Check sheet for the modelled part. Datum: model origin and axes. Units: mm. Face numbers are marked on the shaded views. A direction names the side the tool comes from. Round coordinates to 2 decimals unless told otherwise and drop trailing zeros. Write each loop counter-clockwise with the first axis right and the second up, starting at its lowest first coordinate (ties: lowest second). Pieces come first, ordered by that corner, then holes. Notation, with made-up numbers: (-26, -7.75) -> (-12, -7.75) arc R27 ccw to (-12, 28.25) -> close; hole circle Ø8 at (40, -25). An arc over 180 degrees is marked (long way). Write item = value, one per line.
from build123d import *

# Parameters (mm, degrees)
SKETCH_1_W            = 140
SKETCH_1_H            = 33
EXTRUDE_1_DEPTH       = 3
HOLE_WIZARD_1_D       = 3.5
SKETCH_5_W            = 10
SKETCH_5_H            = 33
EXTRUDE_2_DEPTH       = 31
SKETCH_6_W            = 140
SKETCH_6_H            = 33
EXTRUDE_3_DEPTH       = 3
HOLE_WIZARD_2_D       = 4
HOLE_WIZARD_2_DEPTH   = 3
EXTRUDE_7_DEPTH       = 3
MIRROR_4_COPY_1_DEPTH = 3
EXTRUDE_8_DEPTH       = 3
SKETCH_12_W           = 10
SKETCH_12_H           = 31
CUT_EXTRUDE_1_DEPTH   = 85.528101836
SKETCH_14_W           = 18
SKETCH_14_H           = 3.3
CUT_EXTRUDE_3_DEPTH   = 3
SKETCH_17_W           = 30
SKETCH_17_H           = 15
CUT_EXTRUDE_5_DEPTH   = 5
SKETCH_22_W           = 15
SKETCH_22_H           = 15.5
CUT_EXTRUDE_6_DEPTH   = 3
SKETCH_23_W           = 93
SKETCH_23_H           = 20
CUT_EXTRUDE_7_DEPTH   = 13.5
SKETCH_24_W           = 59
SKETCH_24_H           = 14
CUT_EXTRUDE_8_DEPTH   = 3
SKETCH_26_W           = 59
SKETCH_26_H           = 3
EXTRUDE_9_DEPTH       = 33
SKETCH_27_W           = 1.5
SKETCH_27_H           = 28.5
CUT_EXTRUDE_9_DEPTH   = 3
SKETCH_28_W           = 10
SKETCH_28_H           = 3
EXTRUDE_10_DEPTH      = 3
SKETCH_29_W           = 10
SKETCH_29_H           = 15
CUT_EXTRUDE_10_DEPTH  = 3
SKETCH_30_W           = 4
SKETCH_30_H           = 11
EXTRUDE_11_DEPTH      = 3
CUT_EXTRUDE_11_REACH  = 77.507
SKETCH_31_W           = 7
SKETCH_31_H           = 11
SKETCH_35_W           = 5
SKETCH_35_H           = 11
CUT_EXTRUDE_12_DEPTH  = 13.5
HOLE_WIZARD_3_D       = 3.3
HOLE_WIZARD_3_DEPTH   = 3


with BuildPart() as part:
    # 草图1 → 凸台-拉伸1 (new body)
    with BuildSketch(Plane(origin=(0, 0, 0), x_dir=(1, 0, 0), z_dir=(0, 1, 0))):
        Rectangle(SKETCH_1_W, SKETCH_1_H)
    extrude(amount=EXTRUDE_1_DEPTH)

    # 孔1 (through all)
    with Locations(Plane(origin=(0, 3, 0), x_dir=(1, 0, 0), z_dir=(0, 1, 0))):
        with Locations((-66.5, 13), (-12.5, 13), (-12.5, -13), (-66.5, -13)):
            hole_wizard_1 = Hole(HOLE_WIZARD_1_D / 2)

    # 镜向1: 孔1 across plane
    add(hole_wizard_1.mirror(Plane.ZY), mode=Mode.SUBTRACT)

    # 草图5 → 凸台-拉伸2 (add)
    with BuildSketch(Plane.XZ):
        with Locations((-44.5, 0)):
            Rectangle(SKETCH_5_W, SKETCH_5_H)
        with Locations((-34.5, 0)):
            Rectangle(SKETCH_5_W, SKETCH_5_H)
        with Locations((34.5, 0)):
            Rectangle(SKETCH_5_W, SKETCH_5_H)
        with Locations((44.5, 0)):
            Rectangle(SKETCH_5_W, SKETCH_5_H)
    extrude(amount=EXTRUDE_2_DEPTH)

    # 草图6 → 凸台-拉伸3 (add)
    with BuildSketch(Plane.XZ.offset(31)):
        Rectangle(SKETCH_6_W, SKETCH_6_H)
    extrude(amount=EXTRUDE_3_DEPTH)

    # 孔2
    with Locations(Plane(origin=(0, -34, 0), x_dir=(-1, 0, 0), z_dir=(0, -1, 0))):
        with Locations((57, 0), (22, 0)):
            hole_wizard_2 = Hole(HOLE_WIZARD_2_D / 2, depth=HOLE_WIZARD_2_DEPTH)

    # 镜向2: 孔2 across plane
    add(hole_wizard_2.mirror(Plane.ZY), mode=Mode.SUBTRACT)

    # 草图10 → 凸台-拉伸7 (add)
    with BuildSketch(Plane.XY.offset(16.5)):
        Polygon((-61.709614661, 0), (-49.5, -15.5), (-49.5, -9.231659865), align=None)
        Polygon((-61.709614661, 0), (-49.5, -9.231659865), (-56.771936106, 0), align=None)
        Polygon((-49.5, -15.5), (-70, -31), (-61.709614661, -31), (-49.5, -21.768340135), align=None)
    extrude_7 = extrude(amount=-EXTRUDE_7_DEPTH)

    # 镜向3: 凸台-拉伸7 across plane
    add(extrude_7.mirror(Plane.XY))

    # 镜向4: 凸台-拉伸7 across plane
    add(extrude_7.mirror(Plane.ZY))

    # 镜向4 copy 1 sketch → 镜向4 copy 1 (add)
    with BuildSketch(Plane(origin=(0, 0, -16.5), x_dir=(-1, 0, 0), z_dir=(0, 0, -1))):
        Polygon((-61.709614661, 0), (-49.5, -15.5), (-49.5, -9.231659865), align=None)
        Polygon((-61.709614661, 0), (-49.5, -9.231659865), (-56.771936106, 0), align=None)
        Polygon((-49.5, -15.5), (-70, -31), (-61.709614661, -31), (-49.5, -21.768340135), align=None)
    extrude(amount=-MIRROR_4_COPY_1_DEPTH)

    # 草图11 → 凸台-拉伸8 (add)
    with BuildSketch(Plane.XY.offset(16.5)):
        Polygon((-1.380422804, -1.450613794), (-29.5, -31), (-26.739154392, -31), (0, -2.901227588), align=None)
        Polygon((-29.5, -26.648158618), (-29.5, -31), (-1.380422804, -1.450613794), (0, 0), (-4.141268412, 0), align=None)
        Polygon((0, 0), (-1.380422804, -1.450613794), (0, -2.901227588), (1.380422804, -1.450613794), align=None)
        Polygon((1.380422804, -1.450613794), (0, -2.901227588), (26.739154392, -31), (29.5, -31), align=None)
        Polygon((4.141268412, 0), (0, 0), (1.380422804, -1.450613794), (29.5, -31), (29.5, -26.648158618), align=None)
    extrude_8 = extrude(amount=-EXTRUDE_8_DEPTH)

    # 镜向5: 凸台-拉伸8 across plane
    add(extrude_8.mirror(Plane.XY))

    # 草图12 → 切除-拉伸1 (cut, through all)
    with BuildSketch(Plane.XY.offset(16.5)):
        with Locations((-39.5, -15.5)):
            Rectangle(SKETCH_12_W, SKETCH_12_H)
    cut_extrude_1 = extrude(amount=-CUT_EXTRUDE_1_DEPTH, mode=Mode.SUBTRACT)

    # 镜向6: 切除-拉伸1 across plane
    add(cut_extrude_1.mirror(Plane.ZY), mode=Mode.SUBTRACT)

    # 草图14 → 切除-拉伸3 (cut)
    with BuildSketch(Plane(origin=(0, -31, 0), x_dir=(1, 0, 0), z_dir=(0, 1, 0))):
        with Locations((0, -9.5)):
            Rectangle(SKETCH_14_W, SKETCH_14_H)
    extrude(amount=-CUT_EXTRUDE_3_DEPTH, mode=Mode.SUBTRACT)

    # 草图17 → 切除-拉伸5 (cut)
    with BuildSketch(Plane(origin=(0, 3, 0), x_dir=(1, 0, 0), z_dir=(0, 1, 0))):
        Rectangle(SKETCH_17_W, SKETCH_17_H)
    extrude(amount=-CUT_EXTRUDE_5_DEPTH, mode=Mode.SUBTRACT)

    # 草图22 → 切除-拉伸6 (cut)
    with BuildSketch(Plane.XY.offset(16.5)):
        with Locations((57, -7.75)):
            Rectangle(SKETCH_22_W, SKETCH_22_H)
    extrude(amount=-CUT_EXTRUDE_6_DEPTH, mode=Mode.SUBTRACT)

    # 草图23 → 切除-拉伸7 (cut)
    with BuildSketch(Plane.XY.offset(16.5)):
        with Locations((0, -24)):
            Rectangle(SKETCH_23_W, SKETCH_23_H)
    extrude(amount=-CUT_EXTRUDE_7_DEPTH, mode=Mode.SUBTRACT)

    # 草图24 → 切除-拉伸8 (cut)
    with BuildSketch(Plane.XY.offset(16.5)):
        with Locations((0, -7)):
            Rectangle(SKETCH_24_W, SKETCH_24_H)
    extrude(amount=-CUT_EXTRUDE_8_DEPTH, mode=Mode.SUBTRACT)

    # 草图26 → 凸台-拉伸9 (add)
    with BuildSketch(Plane.XY.offset(16.5)):
        with Locations((0, -12.5)):
            Rectangle(SKETCH_26_W, SKETCH_26_H)
    extrude(amount=-EXTRUDE_9_DEPTH)

    # 草图27 → 切除-拉伸9 (cut)
    with BuildSketch(Plane(origin=(0, -11, 0), x_dir=(1, 0, 0), z_dir=(0, 1, 0))):
        with Locations((-10.75, -0.75)):
            Rectangle(SKETCH_27_W, SKETCH_27_H)
        with Locations((-9.25, -0.75)):
            Rectangle(SKETCH_27_W, SKETCH_27_H)
        with Locations((9.25, -0.75)):
            Rectangle(SKETCH_27_W, SKETCH_27_H)
        with Locations((10.75, -0.75)):
            Rectangle(SKETCH_27_W, SKETCH_27_H)
    extrude(amount=-CUT_EXTRUDE_9_DEPTH, mode=Mode.SUBTRACT)

    # 草图28 → 凸台-拉伸10 (add)
    with BuildSketch(Plane.XY.offset(16.5)):
        with Locations((-39.5, -12.5)):
            Rectangle(SKETCH_28_W, SKETCH_28_H)
        with Locations((39.5, -12.5)):
            Rectangle(SKETCH_28_W, SKETCH_28_H)
    extrude(amount=-EXTRUDE_10_DEPTH)

    # 草图29 → 切除-拉伸10 (cut)
    with BuildSketch(Plane(origin=(0, -11, 0), x_dir=(1, 0, 0), z_dir=(0, 1, 0))):
        Rectangle(SKETCH_29_W, SKETCH_29_H)
    extrude(amount=-CUT_EXTRUDE_10_DEPTH, mode=Mode.SUBTRACT)

    # 草图30 → 凸台-拉伸11 (add)
    with BuildSketch(Plane.XY.offset(16.5)):
        with Locations((0, -5.5)):
            Rectangle(SKETCH_30_W, SKETCH_30_H)
    extrude(amount=-EXTRUDE_11_DEPTH)

    # 草图31 → 切除-拉伸11 (cut, up to next)
    with BuildSketch(Plane(origin=(0, -11, 0), x_dir=(1, 0, 0), z_dir=(0, 1, 0)), mode=Mode.PRIVATE) as cut_extrude_11_sk1:
        with Locations((20.5, -5.5)):
            Rectangle(SKETCH_31_W, SKETCH_31_H)
    cut_extrude_11_tool1 = extrude(cut_extrude_11_sk1.sketch, amount=-CUT_EXTRUDE_11_REACH, mode=Mode.PRIVATE) & part.part
    # 草图31 → 切除-拉伸11 (cut, up to next)
    with BuildSketch(Plane(origin=(0, -11, 0), x_dir=(1, 0, 0), z_dir=(0, 1, 0)), mode=Mode.PRIVATE) as cut_extrude_11_sk2:
        with Locations((20.5, 5.5)):
            Rectangle(SKETCH_31_W, SKETCH_31_H)
    cut_extrude_11_tool2 = extrude(cut_extrude_11_sk2.sketch, amount=-CUT_EXTRUDE_11_REACH, mode=Mode.PRIVATE) & part.part
    add(cut_extrude_11_tool1.solids().sort_by_distance((20.5, -11, 5.5))[0], mode=Mode.SUBTRACT)
    add(cut_extrude_11_tool2.solids().sort_by_distance((20.5, -11, -5.5))[0], mode=Mode.SUBTRACT)

    # 草图35 → 切除-拉伸12 (cut)
    with BuildSketch(Plane.XY.offset(16.5)):
        with Locations((-32, -5.5)):
            Rectangle(SKETCH_35_W, SKETCH_35_H)
    extrude(amount=-CUT_EXTRUDE_12_DEPTH, mode=Mode.SUBTRACT)

    # 孔3
    with Locations(Plane(origin=(0, 3, 0), x_dir=(1, 0, 0), z_dir=(0, 1, 0))):
        with Locations((57, -12.25), (-31, -12.25)):
            Hole(HOLE_WIZARD_3_D / 2, depth=HOLE_WIZARD_3_DEPTH)


solid = part.part
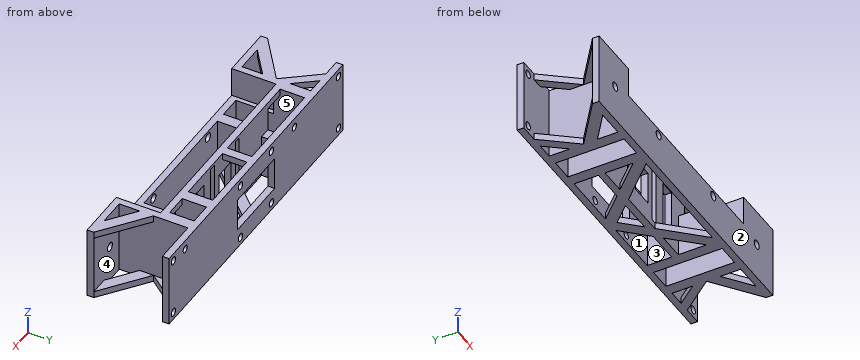
(1) Release check for a two-part mould opening along X. For the marked faces 1 and 2 record: pulls with the +X half, pulls with the -X half, needs draft (parallel to the pull), parting line crosses it, or undercut.
Worked answers:
face_1 = undercut
face_2 = needs draft
(2) Sectioned sample at B-B on z = 0. Count the separate pieces of the cut face and the enclosed holes in it, then the cut area to 3 significant figures.
Worked answers:
separate_pieces = 8
enclosed_holes = 2
area = 1,430 mm²
(3) Access from +Z, -Z, +X, -X, +Y, -Y to the whole of each face (thin tool, end or side, straight path). Record for the marked faces 3, 4 and 5.
Worked answers:
face_3 = +Z, -Z
face_4 = none
face_5 = -Z
(4) Go/stop test with flat-tipped pins: P1, Ø10, axis at y = -13.5, z = 12.5, coming from the +X side; P2, Ø3.5, axis at y = -6, z = -7.5, coming from the -X side; P3, Ø12, axis at y = -11, z = 9, coming from the +X side. Record where each tip stops, or that it passes through.
Worked answers:
P1 = 53.33
P2 = -49.5
P3 = 49.5
(5) Material ranges on L1, parallel to X at y = -29.5, z = -6; L2, parallel to X at y = -9, z = 8; L3, parallel to Z at x = -12.5, y = 2.35, recorded low to high. Write a range as [from, to].
Worked answers:
L1 = [-49.5, -44.5], [-34.5, -29.5], [29.5, 34.5], [44.5, 49.5]
L2 = [-49.5, -44.5], [29.5, 34.5], [44.5, 49.5]
L3 = [-16.5, -14.75], [-11.25, -7.5], [7.5, 11.25], [14.75, 16.5]
(6) Sectioned sample at C-C on x = -66.5. Enter the section's corners in (y, z).
Worked answers:
outline = (-34, -16.5) -> (-28.35, -16.5) -> (-28.35, -13.5) -> (-31, -13.5) -> (-31, 13.5) -> (-28.35, 13.5) -> (-28.35, 16.5) -> (-34, 16.5) -> close; (0, -16.5) -> (3, -16.5) -> (3, -14.75) -> (0, -14.75) -> close; (0, -11.25) -> (3, -11.25) -> (3, 11.25) -> (0, 11.25) -> close; (0, 14.75) -> (3, 14.75) -> (3, 16.5) -> (0, 16.5) -> close
(7) Sectioned sample at A-A on x = -42. Enter the section's corners in (y, z), then the cut area to 4 significant figures.
Worked answers:
outline = (-34, -16.5) -> (-31, -16.5) -> (-31, 3) -> (-34, 3) -> close; (-14, 13.5) -> (-11, 13.5) -> (-11, 16.5) -> (-14, 16.5) -> close; (0, -16.5) -> (3, -16.5) -> (3, 16.5) -> (0, 16.5) -> close
area = 166.5 mm²
(8) Sectioned sample at D-D on x = 22. Enter the section's corners in (y, z).
Worked answers:
outline = (-34, -16.5) -> (-31, -16.5) -> (-31, -2) -> (-34, -2) -> close; (-34, 2) -> (-31, 2) -> (-31, 3) -> (-34, 3) -> close; (-26.02, -16.5) -> (-18.77, -16.5) -> (-18.77, -13.5) -> (-26.02, -13.5) -> close; (-14, -16.5) -> (-11, -16.5) -> (-11, -11) -> (-14, -11) -> close; (-14, 11) -> (-11, 11) -> (-11, 16.5) -> (-14, 16.5) -> close; (0, -16.5) -> (3, -16.5) -> (3, 16.5) -> (0, 16.5) -> close
